For this review, take the finished solid that the model builds, in its own axes (mm). Round coordinates to 2 decimals unless told otherwise and drop trailing zeros. Loops run counter-clockwise (first coordinate to the right, second up) from the corner with the lowest first, then second, coordinate; pieces in that order, holes last.
1) Take a section at A-A (z = -114.3). State the section outline as (x, y) points.
2) Take a section at B-B (x = 19.05). State the section outline as (y, z) points, then the cut area to 3 significant figures.
3) Wall thickness on L1, parallel to X at y = 10.75, z = -65.5; L2, parallel to X at y = 9, z = -66; L3, parallel to X at y = 3.5, z = -12.7: over which ranges is each line inside the solid? List them lowest first.
4) Take a section at D-D (y = 9.5). Give the number of separate pieces and of enclosed holes in the cut face, then the cut area to 3 significant figures.
5) Take a section at C-C (z = -63.5). State the section outline as (x, y) points, then the cut area to 3 significant figures.
6) Insertion check: pin 1 (1 mm diameter, centred on x = 48, y = 3, fed in from +Z); pin 2 (5 mm diameter, centred on x = 61, y = 11, fed in from +Z); pin 3 (1.5 mm diameter, centred on x = 109.5, y = 2, fed in from -Z) (3 decimals). Each pin has a flat end and moves straight along its axis. Give the tip position at first contact, or say it passes through.
```python
from build123d import *

# Parameters (mm, degrees)
SKETCH1_R           = 4.064
BOSS_EXTRUDE1_DEPTH = 12.7
FILLET1_R           = 6.35


with BuildPart() as part:
    # Sketch1 → Boss-Extrude1 (new body)
    with BuildSketch(Plane(origin=(0, 0, 0), x_dir=(1, 0, 0), z_dir=(0, 1, 0))):
        Polygon((0, 0), (0, 127), (38.1, 127), (127, 82.55), (127, 44.45), (38.1, 0), align=None)
        with Locations(Location((19.05, 12.7, 0), (0, 0, 270))):
            Circle(SKETCH1_R, mode=Mode.SUBTRACT)
        with Locations(Location((19.05, 38.1, 0), (0, 0, 270))):
            Circle(SKETCH1_R, mode=Mode.SUBTRACT)
        with Locations(Location((19.05, 63.5, 0), (0, 0, 270))):
            Circle(SKETCH1_R, mode=Mode.SUBTRACT)
        with Locations(Location((19.05, 88.9, 0), (0, 0, 270))):
            Circle(SKETCH1_R, mode=Mode.SUBTRACT)
        with Locations(Location((19.05, 114.3, 0), (0, 0, 270))):
            Circle(SKETCH1_R, mode=Mode.SUBTRACT)
        with Locations(Location((107.95, 63.5, 0), (0, 0, 270))):
            Circle(SKETCH1_R, mode=Mode.SUBTRACT)
        with Locations(Location((82.55, 63.5, 0), (0, 0, 270))):
            Circle(SKETCH1_R, mode=Mode.SUBTRACT)
        with Locations(Location((57.15, 63.5, 0), (0, 0, 270))):
            Circle(SKETCH1_R, mode=Mode.SUBTRACT)
    extrude(amount=BOSS_EXTRUDE1_DEPTH)

    # Fillet1
    fillet1_edges = [part.edges().sort_by_distance(p)[0] for p in [
        (0, 6.35, 0),
        (0, 6.35, -127),
        (38.1, 6.35, -127),
        (127, 6.35, -82.55),
        (127, 6.35, -44.45),
        (38.1, 6.35, 0),
    ]]
    fillet(fillet1_edges, radius=FILLET1_R)


solid = part.part
```
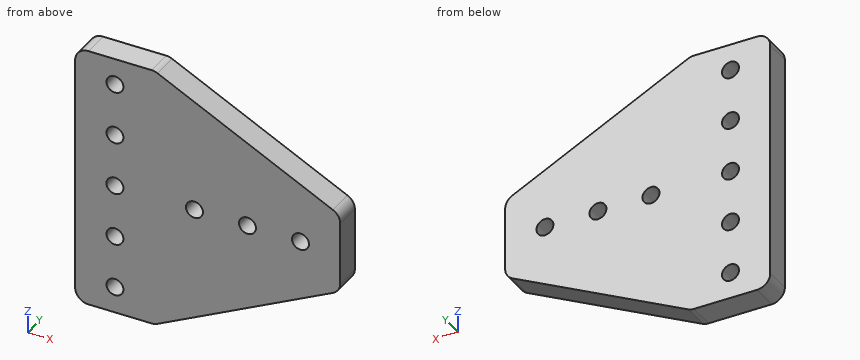
Response:
1. outline: (0, 0) - (14.99, 0) - (14.99, 12.7) - (0, 12.7) - close; (23.11, 0) - (63.5, 0) - (63.5, 12.7) - (23.11, 12.7) - close
2. outline: (0, -127) - (12.7, -127) - (12.7, -118.36) - (0, -118.36) - close; (0, -110.24) - (12.7, -110.24) - (12.7, -92.96) - (0, -92.96) - close; (0, -84.84) - (12.7, -84.84) - (12.7, -67.56) - (0, -67.56) - close; (0, -59.44) - (12.7, -59.44) - (12.7, -42.16) - (0, -42.16) - close; (0, -34.04) - (12.7, -34.04) - (12.7, -16.76) - (0, -16.76) - close; (0, -8.64) - (12.7, -8.64) - (12.7, 0) - (0, 0) - close
2. area: 1,100 mm2
3. L1: x = 0 to 15.51, 22.59 to 53.61, 60.69 to 79.01, 86.09 to 104.41, 111.49 to 127
3. L2: x = 0 to 15.85, 22.25 to 53.95, 60.35 to 79.35, 85.75 to 104.75, 111.15 to 127
3. L3: x = 0 to 14.99, 23.11 to 63.5
4. separate pieces: 1
4. enclosed holes: 8
4. area: 11,700 mm2
5. outline: (0, 0) - (14.99, 0) - (14.99, 12.7) - (0, 12.7) - close; (23.11, 0) - (53.09, 0) - (53.09, 12.7) - (23.11, 12.7) - close; (61.21, 0) - (78.49, 0) - (78.49, 12.7) - (61.21, 12.7) - close; (86.61, 0) - (103.89, 0) - (103.89, 12.7) - (86.61, 12.7) - close; (112.01, 0) - (127, 0) - (127, 12.7) - (112.01, 12.7) - close
5. area: 1,200 mm2
6. pin 1: stops at z = -4.7
6. pin 2: stops at z = -10.2
6. pin 3: stops at z = -91.675
